from build123d import *

# Parameters (mm, degrees)
SKETCH2_W            = 150
SKETCH2_H            = 40
BOSS_EXTRUDE1_DEPTH  = 225
SKETCH3_W            = 140
SKETCH3_H            = 35
CUT_EXTRUDE1_DEPTH   = 50
SKETCH4_W            = 26
SKETCH4_H            = 2
SKETCH4_W_2          = 20
BOSS_EXTRUDE2_DEPTH  = 15
SKETCH6_W            = 10
SKETCH6_H            = 15
CUT_EXTRUDE2_DEPTH   = 15
CUT_EXTRUDE3_DEPTH   = 67
SKETCH9_W            = 10
SKETCH9_H            = 15
CUT_EXTRUDE4_DEPTH   = 67
SKETCH12_W           = 14
SKETCH12_H           = 2
BOSS_EXTRUDE3_DEPTH  = 2.5
FILLET1_R            = 0.5
MIRROR3_START        = 196
MIRROR3_DEPTH        = 14
MIRROR3_START_2      = 15
MIRROR3_2_DEPTH      = 14
MIRROR3_3_DEPTH      = 2
MIRROR3_START_3      = 208
MIRROR3_4_DEPTH      = 2
MIRROR3_5_DEPTH      = 2
MIRROR3_START_4      = 27
MIRROR3_6_DEPTH      = 2
SKETCH16_W           = 32.5
SKETCH16_H           = 11.5
BOSS_EXTRUDE5_DEPTH  = 5
SKETCH17_R           = 1
BOSS_EXTRUDE7_DEPTH  = 25
SKETCH18_W           = 5
SKETCH18_H           = 50
SKETCH18_W_2         = 10
SKETCH18_H_2         = 5
BOSS_EXTRUDE8_DEPTH  = 7.5
SKETCH24_W           = 5.5
SKETCH24_H           = 28
BOSS_EXTRUDE11_DEPTH = 50
SKETCH25_W           = 5
SKETCH25_H           = 28
BOSS_EXTRUDE12_DEPTH = 190
SKETCH26_W           = 5
SKETCH26_H           = 28
BOSS_EXTRUDE13_DEPTH = 190
SKETCH27_R           = 2.55
BOSS_EXTRUDE14_DEPTH = 10
SKETCH29_W           = 10
SKETCH29_H           = 15
CUT_EXTRUDE5_DEPTH   = 19
SKETCH30_W           = 15
SKETCH30_H           = 20
BOSS_EXTRUDE15_DEPTH = 7.5
SKETCH32_W           = 10
SKETCH32_H           = 15
CUT_EXTRUDE6_DEPTH   = 19


# Read off the part's stored shape, not the designer's step: Mirror3
with BuildPart() as part:
    # Sketch2 → Boss-Extrude1 (new body)
    with BuildSketch(Plane.XY):
        Rectangle(SKETCH2_W, SKETCH2_H)
    extrude(amount=BOSS_EXTRUDE1_DEPTH)

    # Sketch3 → Cut-Extrude1 (cut)
    with BuildSketch(Plane.XY.offset(225)):
        Rectangle(SKETCH3_W, SKETCH3_H)
    cut_extrude1 = extrude(amount=-CUT_EXTRUDE1_DEPTH, mode=Mode.SUBTRACT)

    # Sketch4 → Boss-Extrude2 (add)
    with BuildSketch(Plane(origin=(0, -17.5, 0), x_dir=(1, 0, 0), z_dir=(0, 1, 0))):
        Polygon((-42, -196), (-44, -196), (-44, -208), (-44, -210), (-42, -210), align=None)
        with Locations((-57, -209)):
            Rectangle(SKETCH4_W, SKETCH4_H)
        with Locations((-60, -197)):
            Rectangle(SKETCH4_W_2, SKETCH4_H)
        Polygon((70, -210), (70, -208), (44, -208), (44, -196), (42, -196), (42, -210), (44, -210), align=None)
        with Locations((60, -197)):
            Rectangle(SKETCH4_W_2, SKETCH4_H)
    boss_extrude2 = extrude(amount=BOSS_EXTRUDE2_DEPTH)

    # Sketch6 → Cut-Extrude2 (cut)
    with BuildSketch(Plane(origin=(-70, 0, 0), x_dir=(0, 0, -1), z_dir=(1, 0, 0))):
        with Locations((-203, -10)):
            Rectangle(SKETCH6_W, SKETCH6_H)
    cut_extrude2 = extrude(amount=-CUT_EXTRUDE2_DEPTH, mode=Mode.SUBTRACT)

    # Sketch8 → Cut-Extrude3 (cut)
    with BuildSketch(Plane(origin=(0, -17.5, 0), x_dir=(1, 0, 0), z_dir=(0, 1, 0))):
        with BuildLine():
            Line((-64.5, -179.5), (-49.5, -179.5))
            ThreePointArc((-49.5, -179.5), (-46, -183), (-49.5, -186.5))
            Line((-49.5, -186.5), (-64.5, -186.5))
            ThreePointArc((-64.5, -186.5), (-68, -183), (-64.5, -179.5))
        make_face()
        with BuildLine():
            Line((64.5, -179.5), (49.5, -179.5))
            ThreePointArc((49.5, -179.5), (46, -183), (49.5, -186.5))
            Line((49.5, -186.5), (64.5, -186.5))
            ThreePointArc((64.5, -186.5), (68, -183), (64.5, -179.5))
        make_face()
    cut_extrude3 = extrude(amount=CUT_EXTRUDE3_DEPTH, mode=Mode.SUBTRACT)

    # Sketch9 → Cut-Extrude4 (cut)
    with BuildSketch(Plane.ZY.offset(-70)):
        with Locations((203, -10)):
            Rectangle(SKETCH9_W, SKETCH9_H)
    cut_extrude4 = extrude(amount=-CUT_EXTRUDE4_DEPTH, mode=Mode.SUBTRACT)

    # Mirror1: Cut-Extrude1, Boss-Extrude2, Cut-Extrude2, Cut-Extrude3, Cut-Extrude4 across plane
    add(cut_extrude1.mirror(Plane.XY.offset(112.5)), mode=Mode.SUBTRACT)
    add(boss_extrude2.mirror(Plane.XY.offset(112.5)))
    add(cut_extrude2.mirror(Plane.XY.offset(112.5)), mode=Mode.SUBTRACT)
    add(cut_extrude3.mirror(Plane.XY.offset(112.5)), mode=Mode.SUBTRACT)
    add(cut_extrude4.mirror(Plane.XY.offset(112.5)), mode=Mode.SUBTRACT)

    # Sketch12 → Boss-Extrude3 (add)
    with BuildSketch(Plane.ZY.offset(-70)):
        with Locations((22, -1.5)):
            Rectangle(SKETCH12_W, SKETCH12_H)
    extrude(amount=BOSS_EXTRUDE3_DEPTH)

    # Fillet1
    fillet1_edges = [part.edges().sort_by_distance(p)[0] for p in [
        (67.5, -2.5, 22),
    ]]
    fillet(fillet1_edges, radius=FILLET1_R)

    # Mirror3 outline → Mirror3 (add)
    with BuildSketch(Plane.XY.offset(MIRROR3_START)):
        with BuildLine():
            Line((-70, -2.5), (-68, -2.5))
            ThreePointArc((-68, -2.5), (-67.646446609, -2.353553391), (-67.5, -2))
            Line((-67.5, -2), (-67.5, -0.5))
            Line((-67.5, -0.5), (-70, -0.5))
            Line((-70, -0.5), (-70, -2.5))
        make_face()
        with BuildLine():
            Line((68, -2.5), (70, -2.5))
            Line((70, -2.5), (70, -0.5))
            Line((70, -0.5), (67.5, -0.5))
            Line((67.5, -0.5), (67.5, -2))
            ThreePointArc((67.5, -2), (67.646446609, -2.353553391), (68, -2.5))
        make_face()
    extrude(amount=MIRROR3_DEPTH)

    # Mirror3 2 outline → Mirror3 2 (add)
    with BuildSketch(Plane.XY.offset(MIRROR3_START_2)):
        with BuildLine():
            Line((-70, -2.5), (-68, -2.5))
            ThreePointArc((-68, -2.5), (-67.646446609, -2.353553391), (-67.5, -2))
            Line((-67.5, -2), (-67.5, -0.5))
            Line((-67.5, -0.5), (-70, -0.5))
            Line((-70, -0.5), (-70, -2.5))
        make_face()
    extrude(amount=MIRROR3_2_DEPTH)

    # Mirror3 3 outline → Mirror3 3 (add)
    with BuildSketch(Plane.XY.offset(MIRROR3_START)):
        with BuildLine():
            ThreePointArc((-67.5, -2), (-67.646446609, -2.353553391), (-68, -2.5))
            Line((-68, -2.5), (-67.5, -2.5))
            Line((-67.5, -2.5), (-67.5, -2))
        make_face()
        with BuildLine():
            Line((67.5, -2.5), (68, -2.5))
            ThreePointArc((68, -2.5), (67.646446609, -2.353553391), (67.5, -2))
            Line((67.5, -2), (67.5, -2.5))
        make_face()
    extrude(amount=MIRROR3_3_DEPTH)

    # Mirror3 4 outline → Mirror3 4 (add)
    with BuildSketch(Plane.XY.offset(MIRROR3_START_3)):
        with BuildLine():
            ThreePointArc((-67.5, -2), (-67.646446609, -2.353553391), (-68, -2.5))
            Line((-68, -2.5), (-67.5, -2.5))
            Line((-67.5, -2.5), (-67.5, -2))
        make_face()
        with BuildLine():
            Line((67.5, -2.5), (68, -2.5))
            ThreePointArc((68, -2.5), (67.646446609, -2.353553391), (67.5, -2))
            Line((67.5, -2), (67.5, -2.5))
        make_face()
    extrude(amount=MIRROR3_4_DEPTH)

    # Mirror3 5 outline → Mirror3 5 (add)
    with BuildSketch(Plane.XY.offset(MIRROR3_START_2)):
        with BuildLine():
            ThreePointArc((-67.5, -2), (-67.646446609, -2.353553391), (-68, -2.5))
            Line((-68, -2.5), (-67.5, -2.5))
            Line((-67.5, -2.5), (-67.5, -2))
        make_face()
    extrude(amount=MIRROR3_5_DEPTH)

    # Mirror3 6 outline → Mirror3 6 (add)
    with BuildSketch(Plane.XY.offset(MIRROR3_START_4)):
        with BuildLine():
            ThreePointArc((-67.5, -2), (-67.646446609, -2.353553391), (-68, -2.5))
            Line((-68, -2.5), (-67.5, -2.5))
            Line((-67.5, -2.5), (-67.5, -2))
        make_face()
    extrude(amount=MIRROR3_6_DEPTH)

    # Sketch16 → Boss-Extrude5 (add)
    with BuildSketch(Plane(origin=(-70, 0, 0), x_dir=(0, 0, -1), z_dir=(1, 0, 0))):
        with Locations((16.25, -14.25)):
            Rectangle(SKETCH16_W, SKETCH16_H)
    boss_extrude5 = extrude(amount=-BOSS_EXTRUDE5_DEPTH)

    # Mirror4: Boss-Extrude5 across plane
    add(boss_extrude5.mirror(Plane(origin=(0, 0, 0), x_dir=(0, 0, 1), z_dir=(1, 0, 0))))

    # Sketch17 → Boss-Extrude7 (add)
    with BuildSketch(Plane.ZY.offset(-70)):
        with Locations(Location((-29.5, -14.25, 0), (0, 0, 270))):
            Circle(SKETCH17_R)
        with Locations(Location((-3, -14.25, 0), (0, 0, 270))):
            Circle(SKETCH17_R)
    boss_extrude7 = extrude(amount=BOSS_EXTRUDE7_DEPTH)

    # Mirror5: Boss-Extrude7 across plane
    add(boss_extrude7.mirror(Plane(origin=(0, 0, 0), x_dir=(0, 0, 1), z_dir=(1, 0, 0))))

    # Sketch18 → Boss-Extrude8 (add)
    with BuildSketch(Plane(origin=(0, 20, 0), x_dir=(1, 0, 0), z_dir=(0, 1, 0))):
        with Locations((-67.5, -80.5)):
            Rectangle(SKETCH18_W, SKETCH18_H)
        with Locations((67.5, -144.5)):
            Rectangle(SKETCH18_W, SKETCH18_H)
        with Locations((-30, -172)):
            Rectangle(SKETCH18_W_2, SKETCH18_H_2)
        with Locations((-30, -117)):
            Rectangle(SKETCH18_W_2, SKETCH18_H_2)
        with Locations((30, -108)):
            Rectangle(SKETCH18_W_2, SKETCH18_H_2)
        with Locations((30, -53)):
            Rectangle(SKETCH18_W_2, SKETCH18_H_2)
    extrude(amount=BOSS_EXTRUDE8_DEPTH)

    # Sketch24 → Boss-Extrude11 (add)
    with BuildSketch(Plane.ZY.offset(75)):
        with Locations((84.75, -6)):
            Rectangle(SKETCH24_W, SKETCH24_H)
    boss_extrude11 = extrude(amount=BOSS_EXTRUDE11_DEPTH)

    # Sketch25 → Boss-Extrude12 (add)
    with BuildSketch(Plane(origin=(0, 0, 82), x_dir=(-1, 0, 0), z_dir=(0, 0, -1))):
        with Locations((122.5, -6)):
            Rectangle(SKETCH25_W, SKETCH25_H)
    extrude(amount=BOSS_EXTRUDE12_DEPTH)

    # Mirror12: Boss-Extrude11 across plane
    add(boss_extrude11.mirror(Plane(origin=(0, 0, 0), x_dir=(0, 0, 1), z_dir=(1, 0, 0))))

    # Sketch26 → Boss-Extrude13 (add)
    with BuildSketch(Plane(origin=(0, 0, 82), x_dir=(-1, 0, 0), z_dir=(0, 0, -1))):
        with Locations((-122.5, -6)):
            Rectangle(SKETCH26_W, SKETCH26_H)
    extrude(amount=BOSS_EXTRUDE13_DEPTH)

    # Sketch27 → Boss-Extrude14 (add)
    with BuildSketch(Plane.ZY.offset(-120)):
        with Locations(Location((-100.5, -6, 0), (0, 0, 180))):
            Circle(SKETCH27_R)
    boss_extrude14 = extrude(amount=BOSS_EXTRUDE14_DEPTH)

    # Mirror13: Boss-Extrude14 across plane
    add(boss_extrude14.mirror(Plane(origin=(0, 0, 0), x_dir=(0, 0, 1), z_dir=(1, 0, 0))))

    # Sketch29 → Cut-Extrude5 (cut)
    with BuildSketch(Plane.ZY.offset(125)):
        with Locations((-100.5, -6)):
            Rectangle(SKETCH29_W, SKETCH29_H)
    extrude(amount=-CUT_EXTRUDE5_DEPTH, mode=Mode.SUBTRACT)

    # Sketch30 → Boss-Extrude15 (add)
    with BuildSketch(Plane.ZY.offset(125)):
        with Locations((-100.5, -6)):
            Rectangle(SKETCH30_W, SKETCH30_H)
    extrude(amount=BOSS_EXTRUDE15_DEPTH)

    # Sketch32 → Cut-Extrude6 (cut)
    with BuildSketch(Plane(origin=(-125, 0, 0), x_dir=(0, 0, -1), z_dir=(1, 0, 0))):
        with Locations((100.5, -6)):
            Rectangle(SKETCH32_W, SKETCH32_H)
    extrude(amount=-CUT_EXTRUDE6_DEPTH, mode=Mode.SUBTRACT)


solid = part.part
The listing builds one solid part. Answer for the finished solid, in the listing's coordinates (mm). A direction names the side the tool comes from. Give positions to 0.01 mm unless a question says otherwise; leave off trailing zeros. Write each loop counter-clockwise with the first axis right and the second up, starting at its lowest first coordinate (ties: lowest second). Pieces come first, ordered by that corner, then holes. Notation, with made-up numbers: (75, -7) -> (129, -7) arc R34 cw to (129, 32) -> close; hole circle Ø5 at (4, 2.5). An arc over 180 degrees is marked (long way). One line per question, with ' | ' between items. Start each with the question number.
1. Find the intervals of material crossed by probe 1 along X at (y, z) = (-1.5, 57); probe 2 along X at (y, z) = (-16.5, 183); probe 3 along X at (y, z) = (-9, -87.5), in increasing order.
2. For faces 4 (the flat face through (-30, 24, 169.5)), 5 (the flat face through (-70, 3, 18)), 6 (the flat face through (-42, -10, 203)), determine the directions among +Z, -Z, +X, -X, +Y, -Y from which every point of the face is accessible in a straight line to the end or side of a thin tool.
3. Section B-B (z = 183) is taken. Determine the outline of the cut face in (x, y), plus the area to 3 significant figures.
4. Given pin 1 Ø2 at (x, y) = (-130.5, -10) entering from +Z; pin 2 Ø8 at (x, y) = (29, 25) entering from +Z; pin 3 Ø18.5 at (x, y) = (-61.5, -9) entering from -Z, each flat-ended and moving along its own axis, determine where each tip first touches the part or whether it passes through.
5. For a pull along X with two mould halves and no side action, classify faces 1 (the flat face through (-65, 24, 81)), 2 (the flat face through (70, 3, 18)), 3 (the flat face through (30, 24, 50.5)) as pulls with the +X half, pulls with the -X half, needs draft (parallel to the pull), parting line crosses it, or undercut.
6. Section A-A (z = -12.5) is taken. Determine the outline of the cut face in (x, y).
7. Section C-C (x = -83) is taken. Determine the outline of the cut face in (y, z), plus the area to 3 significant figures.
8. Section D-D (z = 42) is taken. Determine the outline of the cut face in (x, y).
Response values:
1) probe 1: -125 to -120, -75 to 75, 120 to 125 | probe 2: -75 to -70, 70 to 75 | probe 3: -125 to -120, 120 to 125
2) face 4: -X, +Y | face 5: none | face 6: +Z
3) outline: (-75, -20) -> (75, -20) -> (75, 20) -> (68, 20) -> (68, 17.5) -> (70, 17.5) -> (70, -17.5) -> (-70, -17.5) -> (-70, 17.5) -> (-68, 17.5) -> (-68, 20) -> (-75, 20) -> close; (-46, 17.5) -> (46, 17.5) -> (46, 20) -> (-46, 20) -> close | area: 990 mm2
4) pin 1: z = -93 | pin 2: z = 110.5 | pin 3: z = -32.5
5) face 1: pulls with the +X half | face 2: undercut | face 3: needs draft
6) outline: (-125, -20) -> (-120, -20) -> (-120, 8) -> (-125, 8) -> close; (-75, -20) -> (-70, -20) -> (-70, -8.5) -> (-75, -8.5) -> close; (70, -20) -> (75, -20) -> (75, -8.5) -> (70, -8.5) -> close; (120, -20) -> (125, -20) -> (125, 8) -> (120, 8) -> close
7) outline: (-20, 82) -> (8, 82) -> (8, 87.5) -> (-20, 87.5) -> close | area: 154 mm2
8) outline: (-125, -20) -> (-120, -20) -> (-120, 8) -> (-125, 8) -> close; (-75, -20) -> (75, -20) -> (75, 20) -> (68, 20) -> (68, 17.5) -> (70, 17.5) -> (70, -17.5) -> (-70, -17.5) -> (-70, 17.5) -> (-68, 17.5) -> (-68, 20) -> (-75, 20) -> close; (-46, 17.5) -> (46, 17.5) -> (46, 20) -> (-46, 20) -> close; (120, -20) -> (125, -20) -> (125, 8) -> (120, 8) -> close
